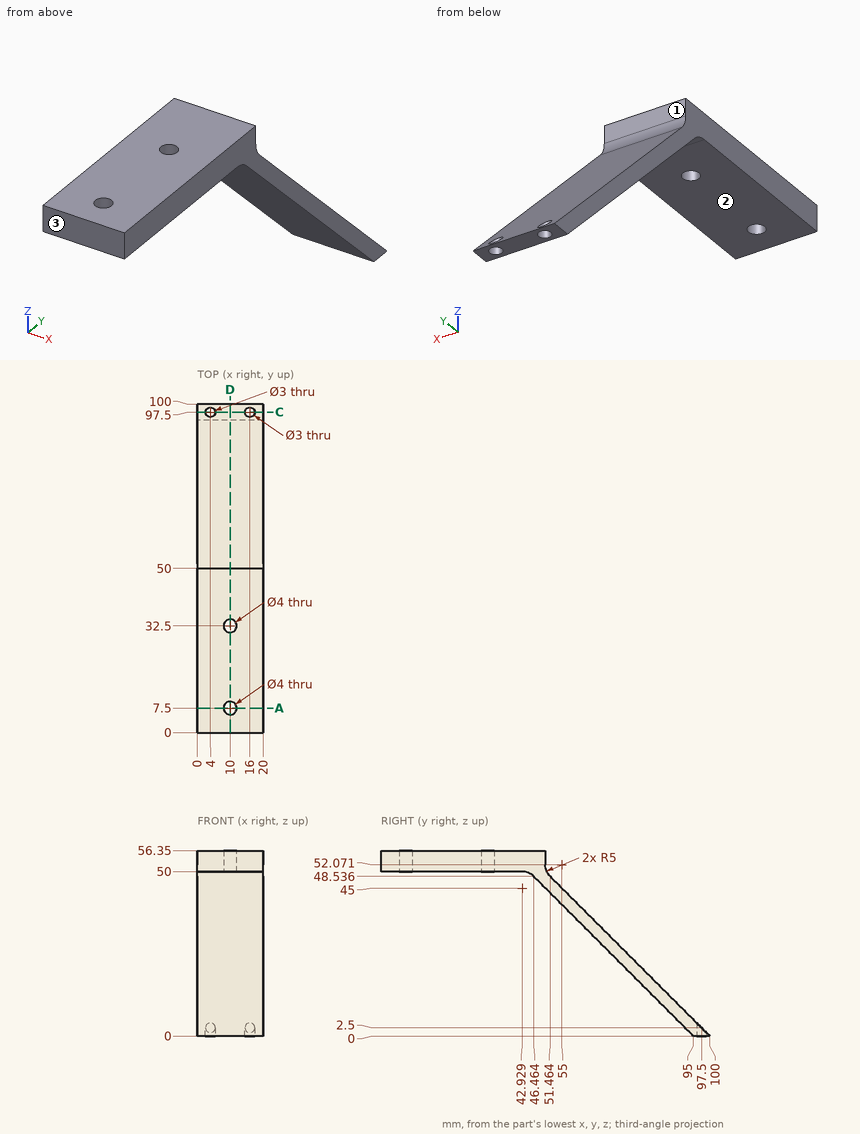
Can you work these out from the drawing? Everything is in mm from the part's minimum corner. A direction names the side the tool comes from. Coordinates: 2 decimals unless noted, no trailing zeros. Loops run counter-clockwise (first coordinate to the right, second up) from the corner with the lowest first, then second, coordinate; pieces in that order, holes last. Notation, with made-up numbers: (-36.75, 80.25) - (5.25, 80.25) arc R21 ccw to (5.25, 110.25) - close; hole circle Ø3 at (-13.5, -2.75). An arc over 180 degrees is marked (long way). Put each result on its own line as item: value. Start each with the question number.
Item 1: If I drill on line 1 along X through (y, z) = (97.5, 1.55); line 2 along Z through (x, y) = (16.75, 15.5); line 3 along X through (y, z) = (7, 53), over which ranges is the centre line in solid material (lowest first)?
Item 2: Suppose I cut it at D-D (x = 10). State how many separate pieces and enclosed holes the cut face has, and give its area (3 significant figures).
Item 3: For pin 1 (10 mm diameter, centred on x = 10, z = 16.5, fed in from +Y); pin 2 (1 mm diameter, centred on x = 8, y = 42, fed in from -Z); pin 3 (3.5 mm diameter, centred on x = 10, y = 32.5, fed in from -Z); pin 4 (1.3 mm diameter, centred on x = 13.5, z = 53.5, fed in from +Y), each with a flat end and sliding along its axis, tell me the tip position at first contact or that it passes through.
Item 4: Suppose I cut it at A-A (y = 7.5). Please give me the cut outline in (x, z).
Item 5: Which directions (+Z, -Z, +X, -X, +Y, -Y) give clear straight access to the entire face, cutting with the end or side of a thin tool? Please do the marked faces 1, 2 and 3.
Item 6: Suppose I cut it at C-C (y = 97.5). Please give me the cut outline in (x, z).
Here are the results:
1. line 1: 0 to 2.5, 5.5 to 14.5, 17.5 to 20
1. line 2: 50 to 56.35
1. line 3: 0 to 8.06, 11.94 to 20
2. separate pieces: 3
2. enclosed holes: 0
2. area: 518 mm²
3. pin 1: y = 88.5
3. pin 2: z = 50
3. pin 3: through
3. pin 4: y = 50
4. outline: (0, 50) - (8, 50) - (8, 56.35) - (0, 56.35) - close; (12, 50) - (20, 50) - (20, 56.35) - (12, 56.35) - close
5. face 1: +Z, +X, -X, +Y
5. face 2: -Z, +X, -X, -Y
5. face 3: +Z, -Z, +X, -X, -Y
6. outline: (0, 0) - (2.5, 0) - (2.5, 2.5) - (0, 2.5) - close; (5.5, 0) - (14.5, 0) - (14.5, 2.5) - (5.5, 2.5) - close; (17.5, 0) - (20, 0) - (20, 2.5) - (17.5, 2.5) - close
